The listing builds one solid part. Answer for the finished solid, in the listing's coordinates (mm). Face numbers are marked on the shaded views. Give positions to 0.01 mm unless a question says otherwise; leave off trailing zeros. Order: outer loops, then holes, each group sorted by start corner. A loop starts at its lowest first (then second) coordinate and runs counter-clockwise, first axis right, second up. Notation, with made-up numbers: (39.25, 82) - (67.25, 82) arc R24 ccw to (67.25, 118) - close; hole circle Ø5 at (20, 20). An arc over 180 degrees is marked (long way). Answer in a Markdown table with one row per item.
from build123d import *

# Parameters (mm, degrees)
F0_W     = 49
F0_H     = 19.05
F1_W     = 48
F1_H     = 19.05
F5_D     = 3.6322
F5_DEPTH = 49.001


with BuildPart() as f2:
    # F0 (on Front) → F2 (revolve)
    with BuildSketch(Plane.XZ):
        with Locations((24.5, -9.525)):
            Rectangle(F0_W, F0_H)
    revolve(axis=Axis((0, 0, -9.525), (0, 0, -1)))

    # F1 (on Right) → F3 (revolve, cut)
    with BuildSketch(Plane.YZ):
        with Locations((-24, -9.525)):
            Rectangle(F1_W, F1_H)
    revolve(axis=Axis((0, 0, -9.525), (0, 0, -1)), mode=Mode.SUBTRACT)

    # F5 (through all, one way)
    with BuildSketch(Plane.XZ):
        with Locations((0, -9.525)):
            Circle(F5_D / 2)
    extrude(amount=-F5_DEPTH, mode=Mode.SUBTRACT)


solid = f2.part
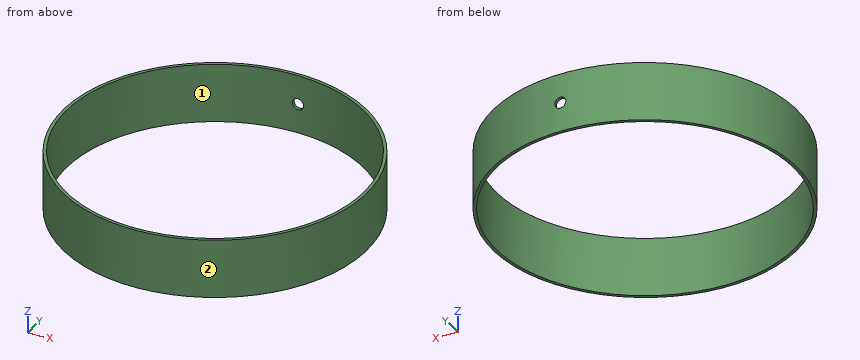
Item 1: Find section D-D on z = -14.25. Write down the section's boundary in (x, y).
Answer block:
| item | result |
|---|---|
| outline | circle Ø98 at (0, 0); hole circle Ø96 at (0, 0) |
Item 2: Find section C-C on x = 25. Write down the section's boundary in (y, z), then the cut area to 3 significant figures.
Answer block:
| item | result |
|---|---|
| outline | (-42.14, -19.05) - (-40.98, -19.05) - (-40.98, 0) - (-42.14, 0) - close; (40.98, -19.05) - (42.14, -19.05) - (42.14, 0) - (40.98, 0) - close |
| area | 44.5 mm² |
Item 3: Find section B-B on x = 0. Write down the section's boundary in (y, z).
Answer block:
| item | result |
|---|---|
| outline | (-49, -19.05) - (-48, -19.05) - (-48, 0) - (-49, 0) - close; (48, -19.05) - (49, -19.05) - (49, -11.34) - (48, -11.34) - close; (48, -7.71) - (49, -7.71) - (49, 0) - (48, 0) - close |
Item 4: Determine the mould class of the marked faces 1 and 2 for opening direction Y: pulls with the +Y half, pulls with the -Y half, needs draft (parallel to the pull), parting line crosses it, or undercut.
Answer block:
| item | result |
|---|---|
| face 1 | undercut |
| face 2 | parting line crosses it |
Item 5: Each of these flat-tipped pins is pushed along its axis until it touches: P1, Ø1, axis at x = 3.5, z = -4, coming from the -Y side; P2, Ø10, axis at y = -12.5, z = -11.5, coming from the +X side; P3, Ø6, axis at x = 4.5, z = -2.5, coming from the +Y side. Where does it stop, or does it pass through?
Answer block:
| item | result |
|---|---|
| P1 | y = -48.91 |
| P2 | x = 48.42 |
| P3 | y = 48.98 |
Item 6: Consider line 1 (Y direction, x = 0, z = -5); line 2 (Y direction, x = 0, z = -8.25). Determine where each line is inside the solid, lowest interval first.
Answer block:
| item | result |
|---|---|
| line 1 | -49 to -48, 48 to 49 |
| line 2 | -49 to -48 |
Item 7: Find section A-A on y = 0. Write down the section's boundary in (x, z).
Answer block:
| item | result |
|---|---|
| outline | (-49, -19.05) - (-48, -19.05) - (-48, 0) - (-49, 0) - close; (48, -19.05) - (49, -19.05) - (49, 0) - (48, 0) - close |
